The listing builds one solid part. Answer for the finished solid, in the listing's coordinates (mm). A direction names the side the tool comes from. Coordinates: 2 decimals unless noted, no trailing zeros. Write each loop counter-clockwise with the first axis right and the second up, starting at its lowest first coordinate (ties: lowest second). Pieces come first, ordered by that corner, then holes.
from build123d import *

# Parameters (mm, degrees)
SKETCH1_W                                            = 120.5
SKETCH1_H                                            = 60
BOSS_EXTRUDE1_DEPTH                                  = 3
SKETCH3_W                                            = 68.5
SKETCH3_H                                            = 28.3
BOSS_EXTRUDE3_DEPTH                                  = 3
BOSS_EXTRUDE2_DEPTH                                  = 10
CSK_FOR_M3_HEX_SOCKET_COUNTERSUNK_CAP_SC_D           = 3.4
CSK_FOR_M3_HEX_SOCKET_COUNTERSUNK_CAP_SC_CSINK_D     = 6.72
CSK_FOR_M3_HEX_SOCKET_COUNTERSUNK_CAP_SC_CSINK_ANGLE = 90
SKETCH6_W                                            = 5
SKETCH6_H                                            = 4
BOSS_EXTRUDE4_DEPTH                                  = 10


with BuildPart() as part:
    # Sketch1 → Boss-Extrude1 (new body)
    with BuildSketch(Plane(origin=(0, 0, 0), x_dir=(1, 0, 0), z_dir=(0, 1, 0))):
        Rectangle(SKETCH1_W, SKETCH1_H)
    extrude(amount=BOSS_EXTRUDE1_DEPTH)

    # Sketch3 → Boss-Extrude3 (add)
    with BuildSketch(Plane.XZ):
        with Locations((0, -44.15)):
            Rectangle(SKETCH3_W, SKETCH3_H)
    extrude(amount=-BOSS_EXTRUDE3_DEPTH)

    # Sketch2 → Boss-Extrude2 (add)
    with BuildSketch(Plane(origin=(0, 3, 0), x_dir=(1, 0, 0), z_dir=(0, 1, 0))):
        Polygon((60.25, 30), (34.25, 30), (34.25, 58.3), (-34.25, 58.3), (-34.25, 30), (-60.25, 30), (-60.25, -30), (60.25, -30), align=None)
        Polygon((-32.25, 28), (-58.25, 28), (-58.25, -28), (58.25, -28), (58.25, 28), (32.25, 28), (32.25, 56.3), (-32.25, 56.3), align=None, mode=Mode.SUBTRACT)
    extrude(amount=BOSS_EXTRUDE2_DEPTH)

    # CSK for M3 Hex Socket Countersunk Cap Screw1 (through all)
    with Locations(Plane(origin=(0, 0, 0), x_dir=(-1, 0, 0), z_dir=(0, -1, 0))):
        with Locations((0, -2.66)):
            CounterSinkHole(CSK_FOR_M3_HEX_SOCKET_COUNTERSUNK_CAP_SC_D / 2, CSK_FOR_M3_HEX_SOCKET_COUNTERSUNK_CAP_SC_CSINK_D / 2, counter_sink_angle=CSK_FOR_M3_HEX_SOCKET_COUNTERSUNK_CAP_SC_CSINK_ANGLE)

    # Sketch6 → Boss-Extrude4 (add)
    with BuildSketch(Plane(origin=(0, 3, 0), x_dir=(1, 0, 0), z_dir=(0, 1, 0))):
        with Locations((-55.75, 26)):
            Rectangle(SKETCH6_W, SKETCH6_H)
    boss_extrude4 = extrude(amount=BOSS_EXTRUDE4_DEPTH)

    # Sketch8 → Ø2.5 (2.5) Diameter Hole1 (revolve, cut)
    with BuildSketch(Plane(origin=(-55.626, 13, -26.296), x_dir=(0, 0, 1), z_dir=(1, 0, 0))):
        Polygon((0, 0), (0, 8.751075774), (1.25, 8), (1.25, 0.125), (1.375, 0), align=None)
    f_2_5_2_5_diameter_hole1 = revolve(axis=Axis((-55.626, 19.35, -26.296), (0, -1, 0)), mode=Mode.SUBTRACT)

    # Mirror1: Boss-Extrude4, Ø2.5 (2.5) Diameter Hole1 across plane
    add(boss_extrude4.mirror(Plane(origin=(0, 0, 0), x_dir=(0, 0, 1), z_dir=(1, 0, 0))))
    add(f_2_5_2_5_diameter_hole1.mirror(Plane(origin=(0, 0, 0), x_dir=(0, 0, 1), z_dir=(1, 0, 0))), mode=Mode.SUBTRACT)


solid = part.part
1. Find the intervals of material crossed by L1, parallel to X at y = 4, z = -36.5; L2, parallel to Z at x = -24, y = 5.5; L3, parallel to X at y = 4.25, z = 15, in increasing order.
Results found:
L1: x = -34.25 to -32.25, 32.25 to 34.25
L2: z = -58.3 to -56.3, 28 to 30
L3: x = -60.25 to -58.25, 58.25 to 60.25
2. Section A-A on x = 0 is taken. Give the vertices of the cut face in (y, z).
Results found:
outline: (0, -58.3) - (13, -58.3) - (13, -56.3) - (3, -56.3) - (3, 0.96) - (1.66, 0.96) - (0, -0.7) - close; (0, 6.02) - (1.66, 4.36) - (3, 4.36) - (3, 28) - (13, 28) - (13, 30) - (0, 30) - close
3. Section C-C on z = 18 is taken. Give the vertices of the cut face in (x, y), then the cut area to 4 significant figures.
Results found:
outline: (-60.25, 0) - (60.25, 0) - (60.25, 13) - (58.25, 13) - (58.25, 3) - (-58.25, 3) - (-58.25, 13) - (-60.25, 13) - close
area: 401.5 mm2
4. A tool of negligible diameter and unlimited length cuts with its end or side. For faces 1 (the flat face through (-60.25, 6, 0)), 2 (the flat face through (-47, 6, -30)), 3 (the flat face through (56, 8, -24)), from which of +Z, -Z, +X, -X, +Y, -Y can it reach the whole face along a straight path? Write none if from no direction.
Results found:
face 1: +Z, -Z, -X, +Y, -Y
face 2: -Z, -X, +Y, -Y
face 3: +Y
5. For a pull along X with two mould halves and no side action, classify faces 4 (the flat face through (34.25, 6, -44)), 5 (the flat face through (-53.25, 8, -26)), 6 (the flat face through (47, 6, -30)), 7 (the flat face through (-34.25, 6, -44)) as pulls with the +X half, pulls with the -X half, needs draft (parallel to the pull), parting line crosses it, or undercut.
Results found:
face 4: pulls with the +X half
face 5: undercut
face 6: needs draft
face 7: pulls with the -X half
6. Section D-D on x = -46 is taken. Give the vertices of the cut face in (y, z), then the cut area to 3 significant figures.
Results found:
outline: (0, -30) - (13, -30) - (13, -28) - (3, -28) - (3, 28) - (13, 28) - (13, 30) - (0, 30) - close
area: 220 mm2
7. Section B-B on z = 2.66 is taken. Give the vertices of the cut face in (x, y).
Results found:
outline: (-60.25, 0) - (-3.36, 0) - (-1.7, 1.66) - (-1.7, 3) - (-58.25, 3) - (-58.25, 13) - (-60.25, 13) - close; (1.7, 1.66) - (3.36, 0) - (60.25, 0) - (60.25, 13) - (58.25, 13) - (58.25, 3) - (1.7, 3) - close
8. Flat-ended cylindrical pins translate along their axes: P1, Ø1, axis at x = -35.5, z = 7, coming from the +Y side; P2, Ø2, axis at x = 55.626, z = -26.296, coming from the +Y side; P3, Ø4, axis at y = 8, z = -44.5, coming from the -X side. Find the tip coordinate at first contact, or state that the pin passes through.
Results found:
P1: stops at y = 3
P2: stops at y = 4.85
P3: stops at x = -34.25
